Geometry check sheet. Reference: the model listing, model coordinates, mm. Face numbers are marked on the shaded views. A direction names the side the tool comes from. Coordinates: 2 decimals unless noted, no trailing zeros. Write each loop counter-clockwise with the first axis right and the second up, starting at its lowest first coordinate (ties: lowest second). Pieces come first, ordered by that corner, then holes. Notation, with made-up numbers: (81, -5) - (125, -5) arc R5 cw to (125, 4) - close; hole circle Ø8 at (26.25, 30.25). An arc over 180 degrees is marked (long way). Answer as a JSON object with one key per item and string values. Group by question number.
from build123d import *

# Parameters (mm, degrees)
SKETCH1_R           = 5
BOSS_EXTRUDE1_DEPTH = 10
SKETCH2_R           = 2.5
BOSS_EXTRUDE2_DEPTH = 24
SKETCH3_R           = 3
CUT_EXTRUDE1_DEPTH  = 5.2
CHAMFER1_SIZE       = 3.2
CHAMFER1_SIZE2      = 1.999581926
SKETCH7_W           = 12.152582876
SKETCH7_H           = 2
CUT_EXTRUDE2_DEPTH  = 6.2
CUT_EXTRUDE3_REACH  = 37.175
SKETCH8_R           = 1


with BuildPart() as part:
    # Sketch1 → Boss-Extrude1 (new body)
    with BuildSketch(Plane.XY):
        Circle(SKETCH1_R)
    extrude(amount=BOSS_EXTRUDE1_DEPTH)

    # Sketch2 → Boss-Extrude2 (add)
    with BuildSketch(Plane.XY.offset(10)):
        Circle(SKETCH2_R)
    extrude(amount=BOSS_EXTRUDE2_DEPTH)

    # Sketch3 → Cut-Extrude1 (cut)
    with BuildSketch(Plane(origin=(0, 0, 0), x_dir=(-1, 0, 0), z_dir=(0, 0, -1))):
        Circle(SKETCH3_R)
    extrude(amount=-CUT_EXTRUDE1_DEPTH, mode=Mode.SUBTRACT)

    # Chamfer1
    chamfer1_edges = [part.edges().sort_by_distance(p)[0] for p in [
        (3, 0, 0),
    ]]
    chamfer1_side = [part.faces().sort_by_distance(p)[0] for p in [
        (3, 0, 2.6),
    ]]
    chamfer(chamfer1_edges, length=CHAMFER1_SIZE, length2=CHAMFER1_SIZE2, reference=chamfer1_side[0])

    # Sketch6 → Cut-Revolve2 (revolve, cut)
    with BuildSketch(Plane(origin=(0, 0, 5.2), x_dir=(-1, 0, 0), z_dir=(0, 0, -1))):
        with BuildLine():
            Line((3, 0), (-3, 0))
            ThreePointArc((-3, 0), (0, -3), (3, 0))
        make_face()
    revolve(axis=Axis((-3, 0, 5.2), (1, 0, 0)), mode=Mode.SUBTRACT)

    # Sketch7 → Cut-Extrude2 (cut)
    with BuildSketch(Plane.XY):
        Rectangle(SKETCH7_W, SKETCH7_H)
    extrude(amount=CUT_EXTRUDE2_DEPTH, mode=Mode.SUBTRACT)

    # Sketch8 → Cut-Extrude3 (cut, up to next)
    with BuildSketch(Plane(origin=(2.5, 0, 0), x_dir=(0, 0, -1), z_dir=(1, 0, 0)), mode=Mode.PRIVATE) as cut_extrude3_sk1:
        with Locations((-21.7, 0)):
            Circle(SKETCH8_R)
    cut_extrude3_tool1 = extrude(cut_extrude3_sk1.sketch, amount=-CUT_EXTRUDE3_REACH, mode=Mode.PRIVATE) & part.part
    add(cut_extrude3_tool1.solids().sort_by_distance((2.5, 0, 21.7))[0], mode=Mode.SUBTRACT)


solid = part.part
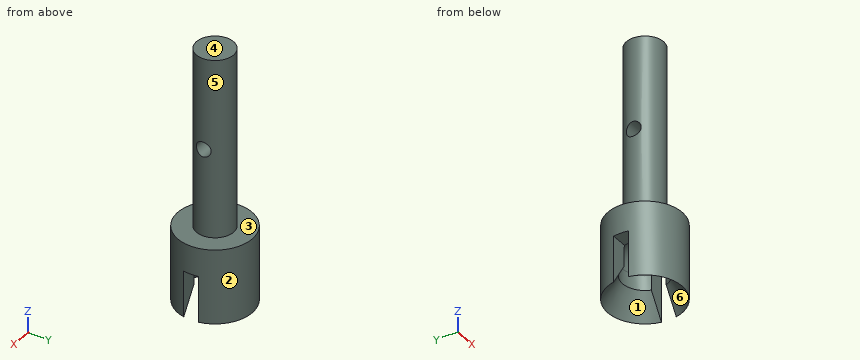
(1) Set-up check for the marked faces 1, 2 and 3: record each of +Z, -Z, +X, -X, +Y, -Y from which the full face is reachable in a straight line by a thin tool's end or side.
(2) Material ranges on L1, parallel to Z at x = 0, y = 0; L2, parallel to Y at x = 1.15, z = 21.7; L3, parallel to X at y = -4, z = 7, recorded low to high. Write a range as [from, to].
(3) Gauge pin test, flat ends, axial feed: pin 1 (1.8 mm diameter, centred on x = -4, z = 4, fed in from -Y); pin 2 (3 mm diameter, centred on x = 2.5, y = 1.5, fed in from +Z); pin 3 (2.5 mm diameter, centred on x = -4.5, z = 3, fed in from +Y); pin 4 (1.5 mm diameter, centred on x = -2, z = 19, fed in from +Y). Record the tip position at first contact, or that the pin passes through.
(4) Draft check along X on the marked faces 4, 5 and 6. Enter one of: +X half, -X half, draft (parallel to the pull), parting line (faces both ways), or undercut.
(5) Section check A-A (y = 0). Record the cut outline in (x, z), and give its area (3 significant figures).
(6) Section check C-C (z = 21.7). Record the cut outline in (x, y), and give its area (3 significant figures).
(7) Section check B-B (z = 9.5). Record the cut outline in (x, y).
Conclusion:
{
 "1": {"face 1": "-Z", "face 2": "+Z, -Z", "face 3": "+Z"},
 "2": {"L1": "z = [8.2, 20.7], [22.7, 34]", "L2": "y = [-2.22, -1], [1, 2.22]", "L3": "x = [-3, 3]"},
 "3": {"pin 1": "stops at y = -3.92", "pin 2": "stops at z = 34", "pin 3": "stops at y = 3.8", "pin 4": "stops at y = 2.17"},
 "4": {"face 4": "draft", "face 5": "parting line", "face 6": "undercut"},
 "5": {"outline": "(-5, 6.2) - (-2.83, 6.2) arc R3 cw to (2.83, 6.2) - (5, 6.2) - (5, 10) - (2.5, 10) - (2.5, 20.7) - (-2.5, 20.7) - (-2.5, 10) - (-5, 10) - close; (-2.5, 22.7) - (2.5, 22.7) - (2.5, 34) - (-2.5, 34) - close", "area": "140 mm^2"},
 "6": {"outline": "(-2.29, -1) arc R2.5 ccw to (2.29, -1) - close; (-2.29, 1) - (2.29, 1) arc R2.5 ccw to start", "area": "9.91 mm^2"},
 "7": {"outline": "circle Ø10 at (0, 0)"}
}
